Could you check a few things on this model? Use its own coordinates, in mm. A direction names the side the tool comes from. Give positions to 0.01 mm unless a question says otherwise; leave off trailing zeros. Order: outer loops, then holes, each group sorted by start corner. A loop starts at its lowest first (then second) coordinate and runs counter-clockwise, first axis right, second up. Notation, with made-up numbers: (10, 15) -> (54, 15) arc R19 ccw to (54, 26) -> close; hole circle Ø7 at (-28.75, -2). An arc over 180 degrees is marked (long way). Answer as CSV lines item,"result". Start each with the question number.
(1) I want a section at A-A (x = 0). Please give me the cut outline in (y, z).
(2) Will these pins go through, and if not, where does the flat tip stop? pin 1 Ø3 at (x, y) = (2, 11.5) entering from +Z; pin 2 Ø2 at (y, z) = (8, -3) entering from -X.
(3) On a 3-axis mill with a long thin cutter (end or side, diameter ignored), from which of +Z, -Z, +X, -X, +Y, -Y can I reach the whole of each face in a straight line? I mean faces 1 (the face through (-0.867, 8.148, -3.905)), 2 (the face through (1, 0, -2)). Say none if no direction works.
(4) I need wall thicknesses on L1, parallel to Z at x = 0, y = -2.25; L2, parallel to Y at x = 1.75, z = 1.75; L3, parallel to Y at x = -1, z = -0.75. Which ranges of each line are inside material? Lowest first, please.
(5) I want a section at C-C (y = -0.25). Please give me the cut outline in (x, z), plus the area to 3 significant figures.
(6) I want a section at D-D (y = 6). Please give me the cut outline in (x, z), plus the area to 3 significant figures.
(7) We'd pull the mould along Z, two halves only. Please class faces 3 (the face through (-1.12, -8.4, -1.03)), 4 (the face through (0, 17, 0)), 5 (the face through (0, -4, -2)), 6 (the face through (0, -0.5, 0)): released by +Z, released by -Z, zero draft, split by the parting line, or undercut.
(8) I want a section at B-B (y = -7). Please give me the cut outline in (x, z), plus the area to 3 significant figures.
```python
from build123d import *

# Parameters (mm, degrees)
F0_R        = 2
F1_DEPTH    = 8
F2_T        = -0.5
F1_FACE_R   = 2
F1_FACE_R_2 = 1.5
F3_DEPTH    = 1
F3_TAPER    = 3
F4_R        = 0.15
F5_R        = 4
F6_DEPTH    = 17
F7_R        = 1
F8_R        = 1.5


with BuildPart() as f1:
    # F0 (on Front) → F1 (new body)
    with BuildSketch(Plane.XZ):
        Circle(F0_R)
    extrude(amount=F1_DEPTH)

    # F2
    f2_openings = [f1.faces().sort_by_distance(p)[0] for p in [
        (0, -8, 0),
    ]]
    offset(amount=F2_T, openings=f2_openings)

    # F1_face (on face) → F3 (join)
    with BuildSketch(Plane.XZ.offset(8)):
        Circle(F1_FACE_R)
        Circle(F1_FACE_R_2, mode=Mode.SUBTRACT)
    extrude(amount=F3_DEPTH, taper=F3_TAPER)

    # F4
    f4_edges = [f1.edges().sort_by_distance(p)[0] for p in [
        (-1.947592, -9, 0),
    ]]
    fillet(f4_edges, radius=F4_R)

    # F5 (on Front) → F6 (join)
    with BuildSketch(Plane.XZ):
        Circle(F5_R)
    extrude(amount=-F6_DEPTH)

    # F7
    f7_edges = [f1.edges().sort_by_distance(p)[0] for p in [
        (-4, 0, 0),
    ]]
    fillet(f7_edges, radius=F7_R)

    # F8
    f8_edges = [f1.edges().sort_by_distance(p)[0] for p in [
        (-4, 17, 0),
    ]]
    fillet(f8_edges, radius=F8_R)


solid = f1.part
```
Final values:
1,outline,"(-9, -1.81) arc R0.15 ccw to (-8.86, -1.96) -> (-8, -2) -> (0, -2) -> (0, -3) arc R1 ccw to (1, -4) -> (15.5, -4) arc R1.5 ccw to (17, -2.5) -> (17, 2.5) arc R1.5 ccw to (15.5, 4) -> (1, 4) arc R1 ccw to (0, 3) -> (0, 2) -> (-8, 2) -> (-8.86, 1.96) arc R0.15 ccw to (-9, 1.81) -> (-9, 1.55) -> (-8, 1.5) -> (-0.5, 1.5) -> (-0.5, -1.5) -> (-8, -1.5) -> (-9, -1.55) -> close"
2,pin 1,"z = 3.97"
2,pin 2,"x = -3.46"
3,face 1,"+Y, -Y"
3,face 2,"-Y"
4,L1,"-2 to -1.5, 1.5 to 2"
4,L2,"0 to 17"
4,L3,"-0.5 to 17"
5,outline,"circle Ø4 at (0, 0)"
5,area,"12.6 mm²"
6,outline,"circle Ø8 at (0, 0)"
6,area,"50.3 mm²"
7,face 3,"undercut"
7,face 4,"zero draft"
7,face 5,"split by the parting line"
7,face 6,"undercut"
8,outline,"circle Ø4 at (0, 0); hole circle Ø3 at (0, 0)"
8,area,"5.50 mm²"
